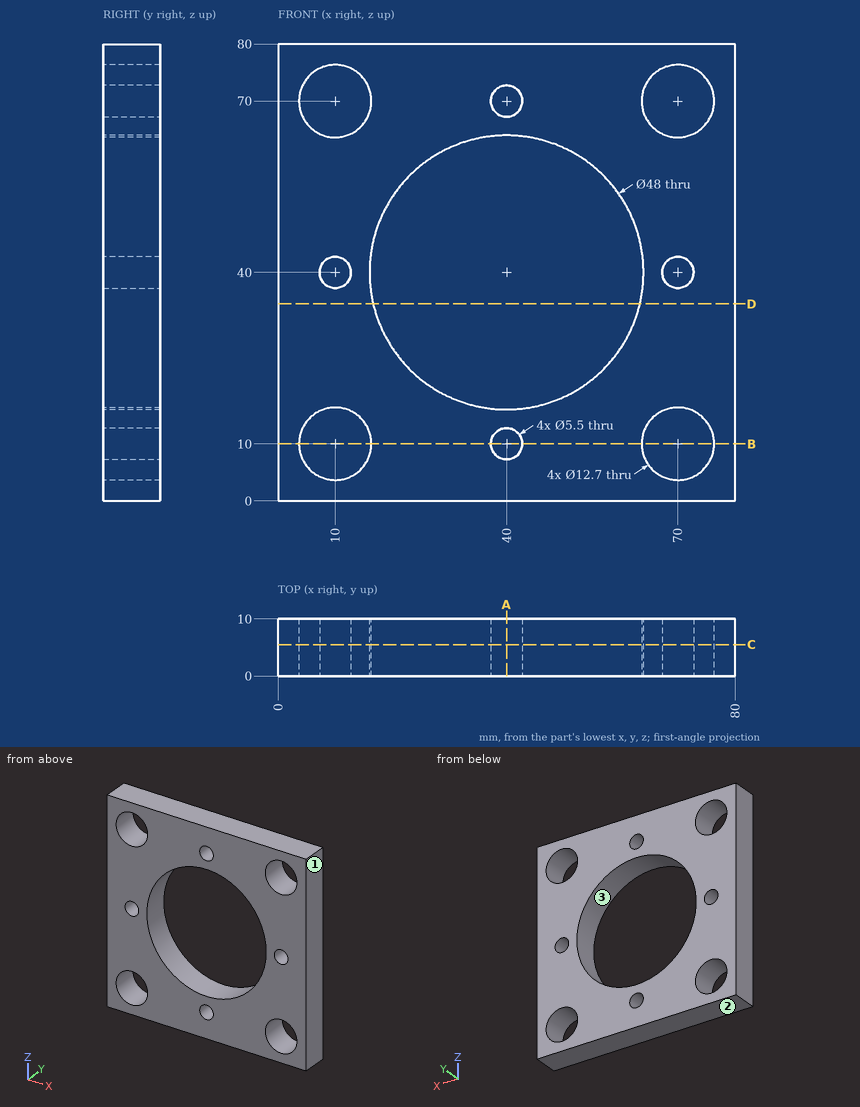
Check sheet for the drawn part. Datum: minimum x, y, z corner. Units: mm. Give positions to 0.01 mm unless a question says otherwise; leave off trailing zeros. Write each loop counter-clockwise with the first axis right and the second up, starting at its lowest first coordinate (ties: lowest second). Pieces come first, ordered by that corner, then holes.
(1) Cross-section at C-C (y = 5.5). State how many separate pieces and enclosed holes the cut face has, plus the area to 3 significant figures.
(2) Cross-section at B-B (z = 10). Enter the section's corners in (x, y).
(3) Gauge pin test, flat end, axial feed: pin 1 (7.5 mm diameter, centred on x = 70, z = 70, fed in from -Y). Record the tip position at first contact, or that the pin passes through.
(4) Cross-section at A-A (x = 40). Enter the section's corners in (y, z), plus the area to 3 significant figures.
(5) Cross-section at D-D (z = 34.5). Enter the section's corners in (x, y).
(6) Mould release check, pull along Z, two halves, no side actions. Record for the marked faces 1, 2 and 3: +Z half, -Z half, draft (parallel to the pull), parting line (faces both ways), or undercut.
(7) Material ranges on line 1 (Z direction, x = 40, y = 3); line 2 (Z direction, x = 70, y = 4.75); line 3 (Z direction, x = 74.5, y = 7.5), recorded low to high.
Worked out:
1. separate pieces: 1
1. enclosed holes: 9
1. area: 3,990 mm2
2. outline: (0, 0) - (3.65, 0) - (3.65, 10) - (0, 10) - close; (16.35, 0) - (37.25, 0) - (37.25, 10) - (16.35, 10) - close; (42.75, 0) - (63.65, 0) - (63.65, 10) - (42.75, 10) - close; (76.35, 0) - (80, 0) - (80, 10) - (76.35, 10) - close
3. pin 1: passes through
4. outline: (0, 0) - (10, 0) - (10, 7.25) - (0, 7.25) - close; (0, 12.75) - (10, 12.75) - (10, 16) - (0, 16) - close; (0, 64) - (10, 64) - (10, 67.25) - (0, 67.25) - close; (0, 72.75) - (10, 72.75) - (10, 80) - (0, 80) - close
4. area: 210 mm2
5. outline: (0, 0) - (16.64, 0) - (16.64, 10) - (0, 10) - close; (63.36, 0) - (80, 0) - (80, 10) - (63.36, 10) - close
6. face 1: draft
6. face 2: -Z half
6. face 3: undercut
7. line 1: z = 0 to 7.25, 12.75 to 16, 64 to 67.25, 72.75 to 80
7. line 2: z = 0 to 3.65, 16.35 to 37.25, 42.75 to 63.65, 76.35 to 80
7. line 3: z = 0 to 5.52, 14.48 to 65.52, 74.48 to 80
